Input: part model. Units: mm. Frame: model coordinates. A direction names the side the tool comes from. Round coordinates to 2 decimals unless told otherwise and drop trailing zeros. Order: outer loops, then holes, each group sorted by start corner. A loop starts at its lowest first (then second) coordinate and runs counter-clockwise, first axis right, second up. Notation, with made-up numbers: M -7,59 L 4,59 A34 cw 4,94 Z; hole C 46,64 d4. An arc over 180 degrees is marked long. One line per question, with ' | ' between items.
```python
from build123d import *

# Parameters (mm, degrees)
SKETCH1_W               = 40
SKETCH1_H               = 90
BOSS_EXTRUDE1_DEPTH     = 20
CUT_EXTRUDE1_DEPTH      = 54.150729064
CUT_EXTRUDE1_DEPTH_BACK = 54.150729064
SKETCH2_R               = 5.1
CUT_EXTRUDE2_DEPTH      = 54.150729064
CUT_EXTRUDE2_DEPTH_BACK = 54.150729064
SKETCH3_R               = 4.5
SKETCH4_R               = 7
CUT_EXTRUDE4_DEPTH      = 9


with BuildPart() as part:
    # Sketch1 → Boss-Extrude1 (new body)
    with BuildSketch(Plane(origin=(0, 0, 0), x_dir=(1, 0, 0), z_dir=(0, 1, 0))):
        Rectangle(SKETCH1_W, SKETCH1_H)
    extrude(amount=BOSS_EXTRUDE1_DEPTH)

    # Sketch2 → Cut-Extrude1 (cut, two sides: drawn at the far end of the back side and taken through both)
    with BuildSketch(Plane(origin=(0, 0, 0), x_dir=(1, 0, 0), z_dir=(0, 1, 0)).offset(-CUT_EXTRUDE1_DEPTH_BACK)):
        with Locations(Location((0, 0, 0), (0, 0, 270))):
            Circle(SKETCH2_R)
    extrude(amount=CUT_EXTRUDE1_DEPTH + CUT_EXTRUDE1_DEPTH_BACK, mode=Mode.SUBTRACT)

    # Sketch3 → Cut-Extrude2 (cut, two sides: drawn at the far end of the back side and taken through both)
    with BuildSketch(Plane(origin=(0, 0, 0), x_dir=(1, 0, 0), z_dir=(0, 1, 0)).offset(-CUT_EXTRUDE2_DEPTH_BACK)):
        with Locations(Location((0, -30, 0), (0, 0, 270))):
            Circle(SKETCH3_R)
        with Locations(Location((0, 30, 0), (0, 0, 270))):
            Circle(SKETCH3_R)
    extrude(amount=CUT_EXTRUDE2_DEPTH + CUT_EXTRUDE2_DEPTH_BACK, mode=Mode.SUBTRACT)

    # Sketch4 → Cut-Extrude4 (cut)
    with BuildSketch(Plane(origin=(0, 0, 0), x_dir=(1, 0, 0), z_dir=(0, 1, 0))):
        with Locations(Location((0, -30, 0), (0, 0, 270))):
            Circle(SKETCH4_R)
        with Locations(Location((0, 30, 0), (0, 0, 270))):
            Circle(SKETCH4_R)
    extrude(amount=CUT_EXTRUDE4_DEPTH, mode=Mode.SUBTRACT)


solid = part.part
```
Item 1: Mould query, pull axis Z, two halves, no side actions, for faces 3 (the flat face through (0, 10, -45)), 4 (the cylindrical face through (1.352, 14.423, 34.292)), 5 (the flat face through (0, 10, 45)), 6 (the flat face through (9, 0, -1)). Classes: +Z half, -Z half, draft (parallel to the pull), parting line (faces both ways), or undercut.
Report:
face 3: -Z half | face 4: undercut | face 5: +Z half | face 6: draft
Item 2: First-contact query: pin 1 (11 mm diameter, centred on x = -3, z = -29.5, fed in from -Y); pin 2 (7 mm diameter, centred on x = 0, z = -30, fed in from -Y); pin 3 (11 mm diameter, centred on x = 0, z = -30, fed in from -Y). Flat tips, straight axial feed; report the tip coordinate or a pass-through.
Report:
pin 1: y = 0 | pin 2: through | pin 3: y = 9
Item 3: Section query B-B, the plane y = 11.5. Return loops of the section in (x, z).
Report:
outline: M -20,-45 L 20,-45 L 20,45 L -20,45 Z; hole C 0,0 d10.2; hole C 0,-30 d9; hole C 0,30 d9
Item 4: Line query: line 1 along Z through (x, y) = (0, 16.5); line 2 along X through (y, z) = (5.75, 30); line 3 along Z through (x, y) = (-1.5, 13.25). Output: solid intervals per line, ascending. Write a range as from..to.
Report:
line 1: -45..-34.5, -25.5..-5.1, 5.1..25.5, 34.5..45 | line 2: -20..-7, 7..20 | line 3: -45..-34.24, -25.76..-4.87, 4.87..25.76, 34.24..45
Item 5: Section query D-D, the plane y = 6.75. Return loops of the section in (x, z).
Report:
outline: M -20,-45 L 20,-45 L 20,45 L -20,45 Z; hole C 0,-30 d14; hole C 0,30 d14; hole C 0,0 d10.2
Item 6: Section query C-C, the plane x = 0. Return loops of the section in (y, z).
Report:
outline: M 0,-45 L 20,-45 L 20,-34.5 L 9,-34.5 L 9,-37 L 0,-37 Z; M 0,-23 L 9,-23 L 9,-25.5 L 20,-25.5 L 20,-5.1 L 0,-5.1 Z; M 0,5.1 L 20,5.1 L 20,25.5 L 9,25.5 L 9,23 L 0,23 Z; M 0,37 L 9,37 L 9,34.5 L 20,34.5 L 20,45 L 0,45 Z
Item 7: Access query for faces 1 (the cylindrical face through (1.532, 9.86, 4.864)), 2 (the cylindrical face through (-2.681, 4.437, -23.534)). Directions: +Z, -Z, +X, -X, +Y, -Y. A direction counts if a zero-diameter tool reaches every point of the face in a straight line with its end or side. Return the directions, or none.
Report:
face 1: +Y, -Y | face 2: -Y
Item 8: Section query A-A, the plane z = 0. Return loops of the section in (x, y).
Report:
outline: M -20,0 L -5.1,0 L -5.1,20 L -20,20 Z; M 5.1,0 L 20,0 L 20,20 L 5.1,20 Z
